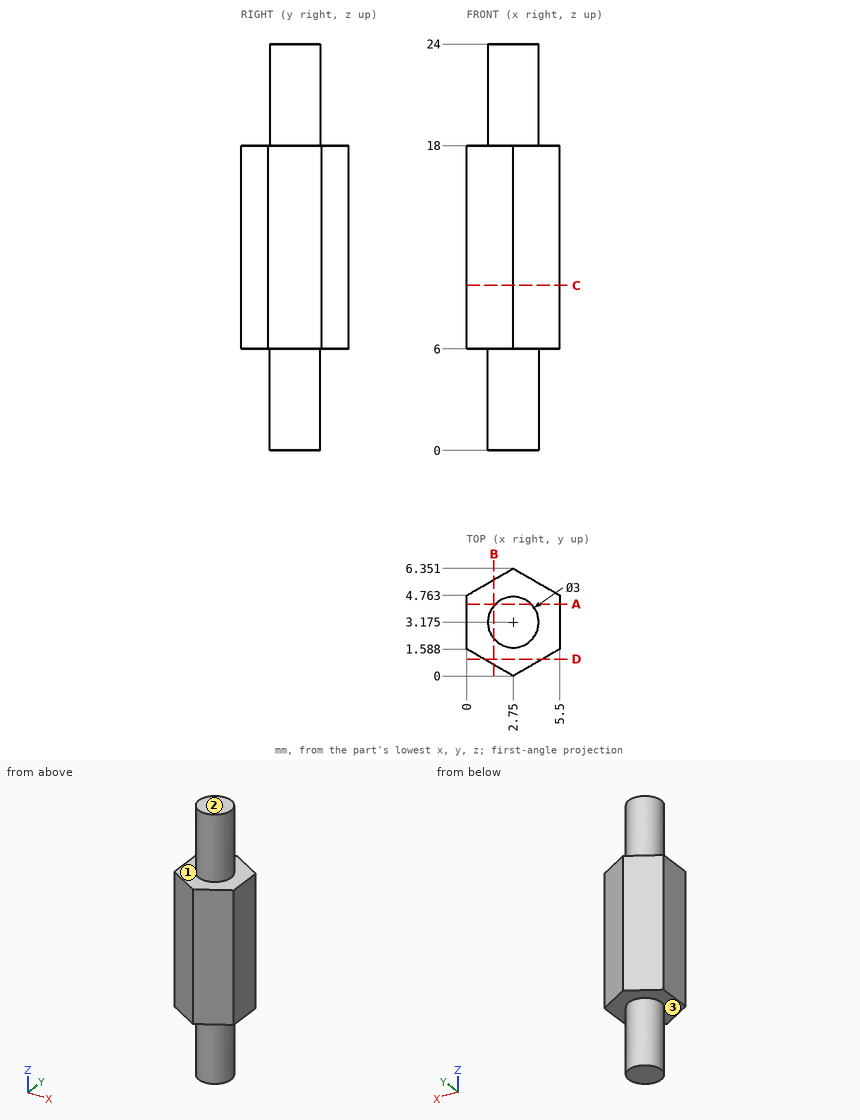
Here's the drawing with two shaded views (mm, measured from the low corner). I have some questions. A direction names the side the tool comes from. Coordinates: 2 decimals unless noted, no trailing zeros. Order: outer loops, then holes, each group sorted by start corner. A loop starts at its lowest first (then second) coordinate and runs counter-clockwise, first axis right, second up. Notation, with made-up numbers: M -32.5,41 L -13.5,41 A16 cw -13.5,70 Z; hole C 89,-15.75 d3. An arc over 180 degrees is marked long. Write item = value, one per line.
(1) Suppose I cut it at A-A on y = 4.25. Please give me the cut outline in (x, z).
Results are:
outline = M 0,6 L 1.7,6 L 1.7,0 L 3.8,0 L 3.8,6 L 5.5,6 L 5.5,18 L 3.8,18 L 3.8,24 L 1.7,24 L 1.7,18 L 0,18 Z
(2) For the marked faces 1, 2 and 3, which set-ups out of +Z, -Z, +X, -X, +Y, -Y let a thin tool reach every point of the face, with its end or its side?
Results are:
face_1 = +Z
face_2 = +Z, +X, -X, +Y, -Y
face_3 = -Z
(3) I need wall thicknesses on line 1 along Z through (x, y) = (2.75, 0.5); line 2 along Y through (x, z) = (4.65, 11.25) (1 decimal); line 3 along Y through (x, z) = (3.9, 1.25) (1 decimal). Which ranges of each line are inside material? Lowest first, please. Write a range as [from, to].
Results are:
line_1 = [6, 18]
line_2 = [1.1, 5.3]
line_3 = [2.2, 4.1]
(4) For pin 1 Ø2 at (x, z) = (4, 11) entering from -Y (1 decimal); pin 2 Ø1 at (y, z) = (1, 9.5) entering from +X; pin 3 Ø1.5 at (x, z) = (3, 21) entering from -Y (1 decimal), each with a flat end and sliding along its axis, tell me the tip position at first contact or that it passes through.
Results are:
pin_1 = 0.1
pin_2 = 5.35
pin_3 = 1.7
(5) Suppose I cut it at D-D on y = 1. Please give me the cut outline in (x, z).
Results are:
outline = M 1.02,6 L 4.48,6 L 4.48,18 L 1.02,18 Z
(6) Suppose I cut it at B-B on x = 1.6. Please give me the cut outline in (y, z).
Results are:
outline = M 0.66,6 L 2.21,6 L 2.21,0 L 4.14,0 L 4.14,6 L 5.69,6 L 5.69,18 L 4.14,18 L 4.14,24 L 2.21,24 L 2.21,18 L 0.66,18 Z
(7) Suppose I cut it at C-C on z = 9.75. Please give me the cut outline in (x, y), plus the area to 3 significant figures.
Results are:
outline = M 0,1.59 L 2.75,0 L 5.5,1.59 L 5.5,4.76 L 2.75,6.35 L 0,4.76 Z
area = 26.2 mm2
